Work out the finished part from the listing and answer in its coordinate system (mm). Face numbers are marked on the shaded views. A direction names the side the tool comes from. Give positions to 0.01 mm unless a question says otherwise; leave off trailing zeros. Order: outer loops, then holes, each group sorted by start corner. A loop starts at its lowest first (then second) coordinate and runs counter-clockwise, first axis right, second up. Notation, with made-up numbers: (2.25, 16) - (38.25, 16) arc R23 ccw to (38.25, 53) - close; hole circle Ø3 at (62, 22). An arc over 180 degrees is marked (long way). Put each result on its own line as item: value.
```python
from build123d import *

# Parameters (mm, degrees)
SKETCH1_R           = 3.937
BOSS_EXTRUDE1_DEPTH = 1.5875
SKETCH2_R           = 2.4511
BOSS_EXTRUDE2_DEPTH = 28.575
CHAMFER1_SIZE       = 0.396875


with BuildPart() as part:
    # Sketch1 → Boss-Extrude1 (new, symmetric)
    with BuildSketch(Plane(origin=(0, 0, 0), x_dir=(1, 0, 0), z_dir=(0, 1, 0))):
        with Locations(Location((0, 0, 0), (0, 0, 270))):
            Circle(SKETCH1_R)
    extrude(amount=BOSS_EXTRUDE1_DEPTH, both=True)

    # Sketch2 → Boss-Extrude2 (add)
    with BuildSketch(Plane.XZ.offset(1.5875)):
        with Locations(Location((0, 0, 0), (0, 0, 270))):
            Circle(SKETCH2_R)
    extrude(amount=BOSS_EXTRUDE2_DEPTH)

    # Chamfer1
    chamfer1_edges = [part.edges().sort_by_distance(p)[0] for p in [
        (0, -1.5875, -3.937),
        (0, 1.5875, -3.937),
        (0, -30.1625, 2.4511),
    ]]
    chamfer(chamfer1_edges, length=CHAMFER1_SIZE)


solid = part.part
```
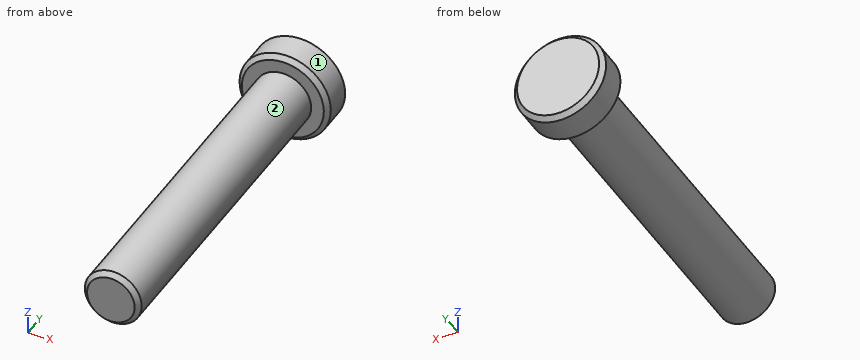
(1) Section A-A, the plane z = 0 is taken. Write down the section's boundary in (x, y), then the cut area to 3 significant figures.
Geometry check:
outline: (-3.94, -1.19) - (-3.54, -1.59) - (-2.45, -1.59) - (-2.45, -29.77) - (-2.05, -30.16) - (2.05, -30.16) - (2.45, -29.77) - (2.45, -1.59) - (3.54, -1.59) - (3.94, -1.19) - (3.94, 1.19) - (3.54, 1.59) - (-3.54, 1.59) - (-3.94, 1.19) - close
area: 165 mm²
(2) Section C-C, the plane y = -19 is taken. Write down the section's boundary in (x, z).
Geometry check:
outline: circle Ø4.9 at (0, 0)
(3) Section B-B, the plane x = 0 is taken. Write down the section's boundary in (y, z), then the cut area to 3 significant figures.
Geometry check:
outline: (-30.16, -2.05) - (-29.77, -2.45) - (-1.59, -2.45) - (-1.59, -3.54) - (-1.19, -3.94) - (1.19, -3.94) - (1.59, -3.54) - (1.59, 3.54) - (1.19, 3.94) - (-1.19, 3.94) - (-1.59, 3.54) - (-1.59, 2.45) - (-29.77, 2.45) - (-30.16, 2.05) - close
area: 165 mm²
(4) A tool of negligible diameter and unlimited length cuts with its end or side. For the marked faces 1 and 2, from which of +Z, -Z, +X, -X, +Y, -Y can it reach the whole face along a straight path? Write none if from no direction.
Geometry check:
face 1: +Y, -Y
face 2: -Y
(5) Given pin 1 (2 mm diameter, centred on y = -26, z = -2, fed in from +X); pin 2 (4 mm diameter, centred on y = -22.5, z = 0, fed in from +X); pin 3 (2 mm diameter, centred on y = -14, z = -2.5, fed in from -X), each flat-ended and moving along its own axis, determine where each tip first touches the part or whether it passes through.
Geometry check:
pin 1: stops at x = 2.24
pin 2: stops at x = 2.45
pin 3: stops at x = -1.94
(6) Straight lines are drawn through the part: line 1 (Y direction, x = 0.75, z = 2.75); line 2 (Z direction, x = -3.25, y = 0.5); line 3 (X direction, y = -22, z = 1.75). For each, find the intervals that lie inside material, in ascending order.
Geometry check:
line 1: y = -1.59 to 1.59
line 2: z = -2.22 to 2.22
line 3: x = -1.72 to 1.72
